Read the model definition and answer for the solid it produces. Units are mm, in the model's axes. A direction names the side the tool comes from. Coordinates: 2 decimals unless noted, no trailing zeros. Write each loop counter-clockwise with the first axis right and the second up, starting at its lowest first coordinate (ties: lowest second). Pieces come first, ordered by that corner, then holes.
(1) The mould has two halves that part along Y. Classify faces 1 (the cylindrical face through (17.75, 28.87, 0.44)), 2 (the flat face through (27, 18, 0)), 3 (the flat face through (14, 20, 8)): +Y half, -Y half, draft (parallel to the pull), parting line (faces both ways), or undercut.
(2) Section D-D on z = 6.25 is taken. Write down the section's boundary in (x, y).
(3) Section B-B on y = 25.5 is taken. Write down the section's boundary in (x, z), then the cut area to 3 significant figures.
(4) Section A-A on z = 0 is taken. Write down the section's boundary in (x, y).
(5) Which of the six approach directions +Z, -Z, +X, -X, +Y, -Y give full straight-line access (tool end or side, diameter ignored) to faces 4 (the flat face through (17, 33, 0)), 5 (the flat face through (18, 9, 0))?
(6) Section C-C on x = 21 is taken. Write down the section's boundary in (y, z).
(7) Given pin 1 (5 mm diameter, centred on y = 11, z = -1, fed in from +X); pin 2 (8 mm diameter, centred on y = 19, z = -0.5, fed in from -X); pin 3 (10 mm diameter, centred on x = 26.5, y = 9.5, fed in from +Z), each flat-ended and moving along its own axis, determine where each tip first touches the part or whether it passes through.
(8) Find the intervals of material crossed by probe 1 along Y at (x, z) = (21, 0); probe 2 along Y at (x, z) = (9, 0); probe 3 along X at (y, z) = (11, 5.25), in increasing order.
from build123d import *

# Parameters (mm, degrees)
EXTRUDE_1_DEPTH    = 8
HOLE_WIZARD_M8_1_D = 6.8


with BuildPart() as part:
    # 스케치1 → 보스-돌출1 (new body, symmetric)
    with BuildSketch(Plane.XY):
        Polygon((0, 0), (0, 33), (35, 33), (35, 18), (18, 18), (18, 0), align=None)
    extrude(amount=EXTRUDE_1_DEPTH, both=True)

    # M8 나사 구멍1 (through all)
    with Locations(Plane.ZY):
        with Locations((0, 25.5)):
            Hole(HOLE_WIZARD_M8_1_D / 2)


solid = part.part
Response:
1. face 1: undercut
1. face 2: -Y half
1. face 3: draft
2. outline: (0, 0) - (18, 0) - (18, 18) - (35, 18) - (35, 33) - (0, 33) - close
3. outline: (0, -8) - (35, -8) - (35, -3.4) - (0, -3.4) - close; (0, 3.4) - (35, 3.4) - (35, 8) - (0, 8) - close
3. area: 322 mm2
4. outline: (0, 0) - (18, 0) - (18, 18) - (35, 18) - (35, 22.1) - (0, 22.1) - close; (0, 28.9) - (35, 28.9) - (35, 33) - (0, 33) - close
5. face 4: +Z, -Z, +X, -X, +Y
5. face 5: +Z, -Z, +X, -Y
6. outline: (18, -8) - (33, -8) - (33, 8) - (18, 8) - close; hole circle Ø6.8 at (25.5, 0)
7. pin 1: stops at x = 18
7. pin 2: stops at x = 0
7. pin 3: passes through
8. probe 1: y = 18 to 22.1, 28.9 to 33
8. probe 2: y = 0 to 22.1, 28.9 to 33
8. probe 3: x = 0 to 18
